from build123d import *

# Parameters (mm, degrees)
SKETCH1_W           = 102.235
SKETCH1_H           = 144.145
SKETCH1_R           = 1.65
BOSS_EXTRUDE1_DEPTH = 10
SKETCH2_R           = 3.25
CUT_EXTRUDE1_DEPTH  = 6
SKETCH4_R           = 2.5
CUT_EXTRUDE2_DEPTH  = 178.002192783
BOSS_EXTRUDE2_START = 5
SKETCH5_W           = 7.63
SKETCH5_H           = 7.63
SKETCH5_R           = 2.5
BOSS_EXTRUDE2_DEPTH = 5
SHELL4_START        = 5
SHELL4_OUTLINE_R    = 8.25
SHELL4_DEPTH        = 5


# Read off the part's stored shape, not the designer's step: Shell4
with BuildPart() as part:
    # Sketch1 → Boss-Extrude1 (new body)
    with BuildSketch(Plane(origin=(0, 0, 0), x_dir=(1, 0, 0), z_dir=(0, 1, 0))):
        with Locations((51.1175, 72.0725)):
            Rectangle(SKETCH1_W, SKETCH1_H)
        with Locations(Location((47.6175, 134.525, 0), (0, 0, 270))):
            Circle(SKETCH1_R, mode=Mode.SUBTRACT)
        with Locations(Location((54.6175, 109.525, 0), (0, 0, 270))):
            Circle(SKETCH1_R, mode=Mode.SUBTRACT)
        with Locations(Location((54.6175, 59.525, 0), (0, 0, 270))):
            Circle(SKETCH1_R, mode=Mode.SUBTRACT)
        with Locations(Location((47.6175, 84.525, 0), (0, 0, 270))):
            Circle(SKETCH1_R, mode=Mode.SUBTRACT)
        with Locations(Location((54.6175, 9.525, 0), (0, 0, 270))):
            Circle(SKETCH1_R, mode=Mode.SUBTRACT)
        with Locations(Location((47.6175, 34.525, 0), (0, 0, 270))):
            Circle(SKETCH1_R, mode=Mode.SUBTRACT)
    extrude(amount=BOSS_EXTRUDE1_DEPTH)

    # Sketch2 → Cut-Extrude1 (cut)
    with BuildSketch(Plane(origin=(0, 10, 0), x_dir=(1, 0, 0), z_dir=(0, 1, 0))):
        with Locations(Location((47.6175, 134.525, 0), (0, 0, 270))):
            Circle(SKETCH2_R)
        with Locations(Location((54.6175, 109.525, 0), (0, 0, 270))):
            Circle(SKETCH2_R)
        with Locations(Location((47.6175, 84.525, 0), (0, 0, 270))):
            Circle(SKETCH2_R)
        with Locations(Location((54.6175, 59.525, 0), (0, 0, 270))):
            Circle(SKETCH2_R)
        with Locations(Location((47.6175, 34.525, 0), (0, 0, 270))):
            Circle(SKETCH2_R)
        with Locations(Location((54.6175, 9.525, 0), (0, 0, 270))):
            Circle(SKETCH2_R)
    extrude(amount=-CUT_EXTRUDE1_DEPTH, mode=Mode.SUBTRACT)

    # Sketch4 → Cut-Extrude2 (cut, through all)
    with BuildSketch(Plane(origin=(0, 10, 0), x_dir=(1, 0, 0), z_dir=(0, 1, 0))):
        with Locations(Location((3.815, 140.33, 0), (0, 0, 270))):
            Circle(SKETCH4_R)
        with Locations(Location((98.42, 140.33, 0), (0, 0, 90))):
            Circle(SKETCH4_R)
        with Locations(Location((98.42, 3.815, 0), (0, 0, 270))):
            Circle(SKETCH4_R)
        with Locations(Location((3.815, 3.815, 0), (0, 0, 90))):
            Circle(SKETCH4_R)
    extrude(amount=-CUT_EXTRUDE2_DEPTH, mode=Mode.SUBTRACT)

    # Sketch5 → Boss-Extrude2 (add)
    # profile 1 of 4: a face of its own
    with BuildSketch(Plane(origin=(0, 10, 0), x_dir=(1, 0, 0), z_dir=(0, 1, 0)).offset(BOSS_EXTRUDE2_START)):
        with Locations((3.815, 140.33)):
            Rectangle(SKETCH5_W, SKETCH5_H)
        with Locations(Location((3.815, 140.33, 0), (0, 0, 270))):
            Circle(SKETCH5_R, mode=Mode.SUBTRACT)
    # profile 2 of 4: a face of its own
    with BuildSketch(Plane(origin=(0, 10, 0), x_dir=(1, 0, 0), z_dir=(0, 1, 0)).offset(BOSS_EXTRUDE2_START)):
        with Locations((98.42, 140.33)):
            Rectangle(SKETCH5_W, SKETCH5_H)
        with Locations(Location((98.42, 140.33, 0), (0, 0, 90))):
            Circle(SKETCH5_R, mode=Mode.SUBTRACT)
    # profile 3 of 4: a face of its own
    with BuildSketch(Plane(origin=(0, 10, 0), x_dir=(1, 0, 0), z_dir=(0, 1, 0)).offset(BOSS_EXTRUDE2_START)):
        with Locations((98.42, 3.815)):
            Rectangle(SKETCH5_W, SKETCH5_H)
        with Locations(Location((98.42, 3.815, 0), (0, 0, 270))):
            Circle(SKETCH5_R, mode=Mode.SUBTRACT)
    # profile 4 of 4: a face of its own
    with BuildSketch(Plane(origin=(0, 10, 0), x_dir=(1, 0, 0), z_dir=(0, 1, 0)).offset(BOSS_EXTRUDE2_START)):
        with Locations((3.815, 3.815)):
            Rectangle(SKETCH5_W, SKETCH5_H)
        with Locations(Location((3.815, 3.815, 0), (0, 0, 90))):
            Circle(SKETCH5_R, mode=Mode.SUBTRACT)
    extrude(amount=-BOSS_EXTRUDE2_DEPTH)

    # Shell4 outline → Shell4 (cut)
    with BuildSketch(Plane(origin=(0, 0, 0), x_dir=(1, 0, 0), z_dir=(0, 1, 0)).offset(SHELL4_START)):
        with BuildLine():
            ThreePointArc((47.719175928, 5), (54.6175, 17.775), (61.515824072, 5))
            Line((61.515824072, 5), (91.01420666, 5))
            ThreePointArc((91.01420666, 5), (93.116699141, 9.118300859), (97.235, 11.22079334))
            Line((97.235, 11.22079334), (97.235, 132.92420666))
            ThreePointArc((97.235, 132.92420666), (93.116699141, 135.026699141), (91.01420666, 139.145))
            Line((91.01420666, 139.145), (54.452564008, 139.145))
            ThreePointArc((54.452564008, 139.145), (47.6175, 126.275), (40.782435992, 139.145))
            Line((40.782435992, 139.145), (11.22079334, 139.145))
            ThreePointArc((11.22079334, 139.145), (9.118300859, 135.026699141), (5, 132.92420666))
            Line((5, 132.92420666), (5, 11.22079334))
            ThreePointArc((5, 11.22079334), (9.118300859, 9.118300859), (11.22079334, 5))
            Line((11.22079334, 5), (47.719175928, 5))
        make_face()
        with Locations((47.6175, 34.525)):
            Circle(SHELL4_OUTLINE_R, mode=Mode.SUBTRACT)
        with Locations((54.6175, 59.525)):
            Circle(SHELL4_OUTLINE_R, mode=Mode.SUBTRACT)
        with Locations((47.6175, 84.525)):
            Circle(SHELL4_OUTLINE_R, mode=Mode.SUBTRACT)
        with Locations((54.6175, 109.525)):
            Circle(SHELL4_OUTLINE_R, mode=Mode.SUBTRACT)
    extrude(amount=SHELL4_DEPTH, mode=Mode.SUBTRACT)


solid = part.part
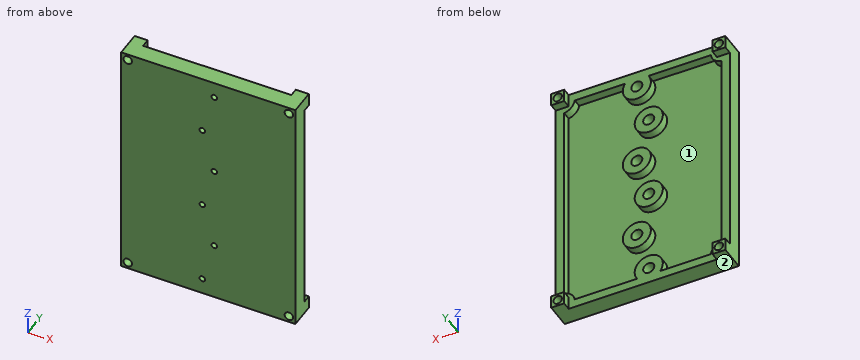
For this review, take the finished solid that the model builds, in its own axes (mm). Face numbers are marked on the shaded views. Round coordinates to 2 decimals unless told otherwise and drop trailing zeros. Loops run counter-clockwise (first coordinate to the right, second up) from the corner with the lowest first, then second, coordinate; pieces in that order, holes last. Notation, with made-up numbers: (-2.75, -23) - (46.25, -23) arc R34 cw to (46.25, 15) - close; hole circle Ø3 at (60, 47.25). An arc over 180 degrees is marked (long way). One line per item, written item: value. Start each with the question number.
Item 1: Take a section at A-A (y = 7.25). State how many separate pieces and enclosed holes the cut face has, plus the area to 3 significant figures.
Item 2: Take a section at B-B (z = -98). Give the boundary of the cut face in (x, y) (3 decimals), plus the area to 3 significant figures.
Item 3: Clearance check with flat-ended pins moving along their axes: pin 1 Ø8 at (x, y) = (32, 12.5) entering from +Z; pin 2 Ø10.5 at (x, z) = (47.62, -134.52) entering from +Y; pin 3 Ø3 at (x, z) = (83.5, -96) entering from +Y; pin 4 Ø5 at (x, z) = (54.62, -59.52) entering from +Y. State where each tip first meets the part, or that it passes through.
Item 4: Take a section at C-C (x = 9.5). Give the boundary of the cut face in (y, z) (3 decimals), plus the area to 3 significant figures.
Item 5: The part is to be moulded in two halves that separate along X. For the marked faces 1 and 2, say which applies: +X half, -X half, draft (parallel to the pull), parting line (faces both ways), or undercut.
Item 6: For L1, parallel to X at y = 5.5, z = -59.5 (3 decimals); L2, parallel to X at y = 4, z = -140.33 (3 decimals); L3, parallel to Z at x = 28, y = 7.75 (3 decimals), list the stretches that pass through material, from the lowest coordinate up.
Answer below:
1. separate pieces: 5
1. enclosed holes: 11
1. area: 3,410 mm2
2. outline: (0, 0) - (102.235, 0) - (102.235, 10) - (97.235, 10) - (97.235, 5) - (5, 5) - (5, 10) - (0, 10) - close
2. area: 561 mm2
3. pin 1: stops at z = 0
3. pin 2: stops at y = 10
3. pin 3: stops at y = 5
3. pin 4: stops at y = 4
4. outline: (0, -144.145) - (10, -144.145) - (10, -135.438) - (5, -135.438) - (5, -8.707) - (10, -8.707) - (10, 0) - (0, 0) - close
4. area: 808 mm2
5. face 1: undercut
5. face 2: draft
6. L1: x = 0 to 5, 46.368 to 51.368, 57.867 to 62.867, 97.235 to 102.235
6. L2: x = 0 to 1.315, 6.315 to 95.92, 100.92 to 102.235
6. L3: z = -144.145 to -139.145, -5 to 0
